from build123d import *

# Parameters (mm, degrees)
SKETCH1_R           = 2.413
SKETCH1_R_2         = 6.35
BOSS_EXTRUDE1_DEPTH = 3.175


with BuildPart() as part:
    # Sketch1 → Boss-Extrude1 (new body)
    with BuildSketch(Plane.XY):
        Polygon((92.594576982, -6.877947448), (92.594576982, 60.126165821), (34.151950775, 60.126165821), (34.151950775, 93.757031287), (-38.373257593, 93.757031287), (-38.373257593, 60.126165821), (-96.8158838, 60.126165821), (-96.8158838, -6.877947448), (-96.8158838, -40.590224659), (-88.470653409, -40.590224659), (-88.470653409, -15.190224659), (-59.260653409, -15.190224659), (-59.260653409, -29.792684659), (55.039346591, -29.792684659), (55.039346591, -15.190224659), (84.249346591, -15.190224659), (84.249346591, -40.590224659), (92.594576982, -40.590224659), align=None)
        with Locations((48.689346591, -24.567904659)):
            Circle(SKETCH1_R, mode=Mode.SUBTRACT)
        with Locations((28.322015094, -24.567904659)):
            Circle(SKETCH1_R, mode=Mode.SUBTRACT)
        with Locations((-32.543321912, -24.567904659)):
            Circle(SKETCH1_R, mode=Mode.SUBTRACT)
        with Locations((-52.910653409, -24.567904659)):
            Circle(SKETCH1_R, mode=Mode.SUBTRACT)
        with Locations((-2.110653409, 69.892524061)):
            Circle(SKETCH1_R_2, mode=Mode.SUBTRACT)
    extrude(amount=BOSS_EXTRUDE1_DEPTH)


solid = part.part
Could you check a few things on this model? Use its own coordinates, in mm. Give positions to 0.01 mm unless a question says otherwise; leave off trailing zeros. Order: outer loops, then holes, each group sorted by start corner. A loop starts at its lowest first (then second) coordinate and runs counter-clockwise, first axis right, second up.
1. Will these pins go through, and if not, where does the flat tip stop? P1, Ø1, axis at x = 63, z = 1.5, coming from the +Y side; P2, Ø1.5, axis at y = 64.5, z = 2.5, coming from the +X side; P3, Ø1.6, axis at x = -76.5, z = 2, coming from the -Y side; P4, Ø4.5, axis at x = -52.91, y = -24.57, coming from the -Z side.
2. Suppose I cut it at B-B (x = -26.5). List the corners of the cut face in (y, z) for me (3 decimals), plus the area to 3 significant figures.
3. We'd pull the mould along Y, two halves only. Please class faces 1 (the cylindrical face through (48.166, -26.924, 1.565)), 2 (the flat face through (-3, 28, 0)), 3 (the cylindrical face through (-30.314, -25.492, 1.565)): pulls with the +Y half, pulls with the -Y half, needs draft (parallel to the pull), parting line crosses it, or undercut.
4. Suppose I cut it at C-C (y = 84). List the corners of the cut face in (x, z) for me (3 decimals).
5. Suppose I cut it at A-A (z = 0.5). List the corners of the cut face in (x, y) for me.
6. I need wall thicknesses on L1, parallel to X at y = -32.5, z = 2.45; L2, parallel to Y at x = -16, z = 0.9; L3, parallel to Y at x = 59, z = 0.6. Which ranges of each line are inside material? Lowest first, please.
Solved:
1. P1: stops at y = 60.13
1. P2: stops at x = 34.15
1. P3: stops at y = -15.19
1. P4: passes through
2. outline: (-29.793, 0) - (93.757, 0) - (93.757, 3.175) - (-29.793, 3.175) - close
2. area: 392 mm2
3. face 1: undercut
3. face 2: needs draft
3. face 3: undercut
4. outline: (-38.373, 0) - (34.152, 0) - (34.152, 3.175) - (-38.373, 3.175) - close
5. outline: (-96.82, -40.59) - (-88.47, -40.59) - (-88.47, -15.19) - (-59.26, -15.19) - (-59.26, -29.79) - (55.04, -29.79) - (55.04, -15.19) - (84.25, -15.19) - (84.25, -40.59) - (92.59, -40.59) - (92.59, 60.13) - (34.15, 60.13) - (34.15, 93.76) - (-38.37, 93.76) - (-38.37, 60.13) - (-96.82, 60.13) - close; hole circle Ø4.83 at (-52.91, -24.57); hole circle Ø4.83 at (-32.54, -24.57); hole circle Ø12.7 at (-2.11, 69.89); hole circle Ø4.83 at (28.32, -24.57); hole circle Ø4.83 at (48.69, -24.57)
6. L1: x = -96.82 to -88.47, 84.25 to 92.59
6. L2: y = -29.79 to 93.76
6. L3: y = -15.19 to 60.13
